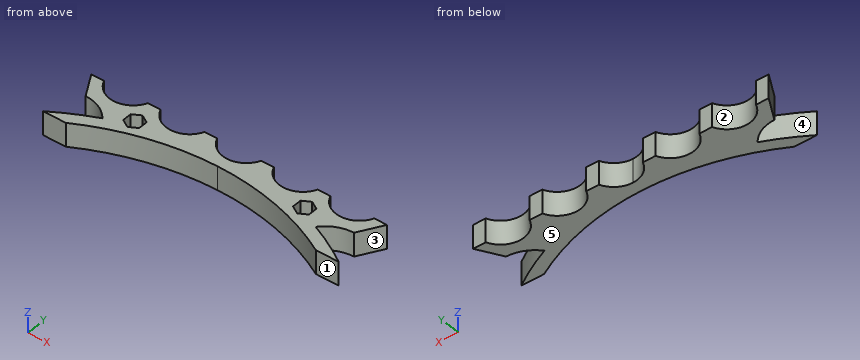
```python
from build123d import *

# Parameters (mm, degrees)
PAD_DEPTH    = 8
POCKET_DEPTH = 6


with BuildPart() as part:
    # Sketch → Pad (new body)
    with BuildSketch(Plane.XY):
        with BuildLine():
            Line((-42.300512, 0), (-50, 0))
            ThreePointArc((-36.046862, 7.541232), (-43.188345, 4.075748), (-50, 0))
            ThreePointArc((-36.046862, 7.541232), (-40.208906, 10.828084), (-45.381198, 12))
            Line((-50, 20), (-45.381198, 12))
            Line((-45.693664, 20), (-50, 20))
            ThreePointArc((-45.693664, 20), (-38.277466, 15), (-30.861267, 20))
            Line((-30.861267, 20), (-26.554931, 20))
            ThreePointArc((-26.554931, 20), (-19.138733, 15), (-11.722534, 20))
            Line((-11.722534, 20), (-7.416198, 20))
            ThreePointArc((-7.416198, 20), (-4.472136, 16.36675), (0, 15))
            Line((0, 11), (0, 15))
            ThreePointArc((0, 11), (-21.85368, 8.205018), (-42.300512, 0))
        make_face()
    pad = extrude(amount=PAD_DEPTH)

    # Mirrored: Pad across Sketch V_Axis
    add(pad.mirror(Plane(origin=(0, 0, 0), x_dir=(0, 0, 1), z_dir=(1, 0, 0))))

    # Sketch001 → Pocket (cut)
    with BuildSketch(Plane.XY.offset(8)):
        Polygon((-28.708099, 15.117691), (-31.408099, 13.558846), (-31.408099, 10.441154), (-28.708099, 8.882309), (-26.008099, 10.441154), (-26.008099, 13.558846), align=None)
    pocket = extrude(amount=-POCKET_DEPTH, mode=Mode.SUBTRACT)

    # Mirrored001: Pocket across Sketch001 V_Axis
    add(pocket.mirror(Plane(origin=(0, 0, 8), x_dir=(0, 0, 1), z_dir=(1, 0, 0))), mode=Mode.SUBTRACT)


solid = part.part
```
Work out the finished part from the listing and answer in its coordinate system (mm). Face numbers are marked on the shaded views. A direction names the side the tool comes from. Round coordinates to 2 decimals unless told otherwise and drop trailing zeros. Loops run counter-clockwise (first coordinate to the right, second up) from the corner with the lowest first, then second, coordinate; pieces in that order, holes last. Notation, with made-up numbers: M 54.5,-15 L 83.5,-15 A24 cw 83.5,14 Z; hole C 26,57.5 d9. An arc over 180 degrees is marked long. One line per question, with ' | ' between items.
Q1. Find section A-A, the plane z = 4.5. State how many separate pieces and enclosed holes the cut face has, then the cut area to 3 significant figures.
Conclusion:
separate pieces: 1 | enclosed holes: 2 | area: 818 mm2
Q2. The mould has two halves that part along X. Classify the marked faces 1, 2 and 3: +X half, -X half, draft (parallel to the pull), parting line (faces both ways), or undercut.
Conclusion:
face 1: draft | face 2: undercut | face 3: +X half
Q3. Consider line 1 along Y through (x, z) = (-28.5, 6); line 2 along Y through (x, z) = (19, 6.5); line 3 along X through (y, z) = (15.75, 7.25). Determine where each line is inside the solid, lowest interval first. Write a range as from..to.
Conclusion:
line 1: y = 6.19..9, 15..20 | line 2: y = 8.9..15 | line 3: x = -47.55..-41.66, -34.9..-22.52, -15.76..-3.38, 3.38..15.76, 22.52..34.9, 41.66..47.55
Q4. Find section B-B, the plane y = 16.75. Give the vertices of the cut face in (x, z).
Conclusion:
outline: M -48.12,0 L -43.27,0 L -43.27,8 L -48.12,8 Z; M -33.28,0 L -24.13,0 L -24.13,8 L -33.28,8 Z; M -14.14,0 L -4.99,0 L -4.99,8 L -14.14,8 Z; M 4.99,0 L 14.14,0 L 14.14,8 L 4.99,8 Z; M 24.13,0 L 33.28,0 L 33.28,8 L 24.13,8 Z; M 43.27,0 L 48.12,0 L 48.12,8 L 43.27,8 Z
Q5. A tool of negligible diameter and unlimited length cuts with its end or side. For the marked faces 4 and 5, from which of +Z, -Z, +X, -X, +Y, -Y can it reach the whole face along a straight path? Write none if from no direction.
Conclusion:
face 4: +Z, -Z, -X | face 5: -Z, +X, -X, +Y, -Y
Q6. Find section D-D, the plane y = 2. Give the vertices of the cut face in (x, z), then the cut area to 3 significant figures.
Conclusion:
outline: M -46.83,0 L -38.5,0 L -38.5,8 L -46.83,8 Z; M 38.5,0 L 46.83,0 L 46.83,8 L 38.5,8 Z | area: 133 mm2
Q7. Find section C-C, the plane x = -44. Give the vertices of the cut face in (y, z).
Conclusion:
outline: M 0,0 L 3.63,0 L 3.63,8 L 0,8 Z; M 11.92,0 L 17.41,0 L 17.41,8 L 11.92,8 Z
Q8. Each of these flat-tipped pins is pushed along its axis until it touches: pin 1 Ø2 at (y, z) = (12, 5) entering from -X; pin 2 Ø3.5 at (y, z) = (12.5, 4) entering from -X; pin 3 Ø2 at (x, z) = (-37.5, 2) entering from -Y. Where does it stop, or does it pass through?
Conclusion:
pin 1: stops at x = -45.96 | pin 2: stops at x = -46.68 | pin 3: stops at y = 2
